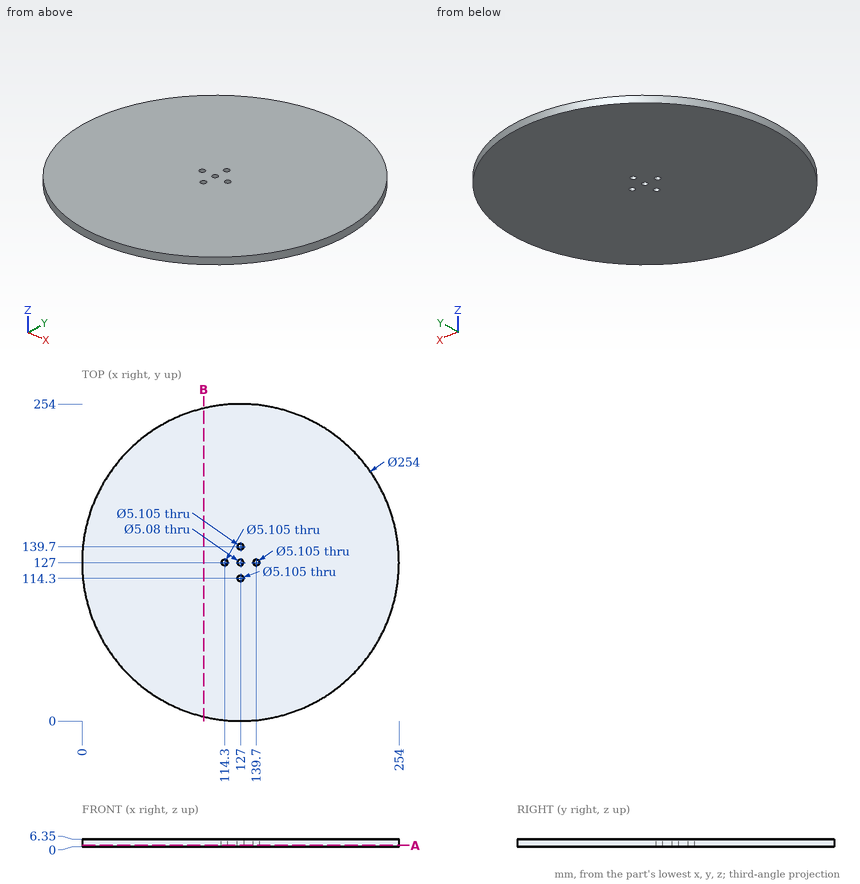
Study the drawing (mm; zero at the part's minimum x, y, z) and answer. Coordinates: 2 decimals unless noted, no trailing zeros. Loops run counter-clockwise (first coordinate to the right, second up) from the corner with the lowest first, then second, coordinate; pieces in that order, holes last. Notation, with made-up numbers: M 57,20 L 83,20 A10 ccw 83,31 Z; hole C 30,42 d1. An arc over 180 degrees is marked long. Answer in a Markdown table with one row per item.
1) Find section A-A (z = 1.25). Determine the outline of the cut face in (x, y) (1 decimal).
Answers below:
| item | result |
|---|---|
| outline | C 127,127 d254; hole C 114.3,127 d5.1; hole C 127,114.3 d5.1; hole C 127,139.7 d5.1; hole C 127,127 d5.1; hole C 139.7,127 d5.1 |
2) Given pin 1 (2 mm diameter, centred on y = 85, z = 4.5, fed in from -X); pin 2 (1 mm diameter, centred on x = 29.5, z = 4.5, fed in from -Y) (1 decimal); pin 3 (3 mm diameter, centred on y = 75, z = 2.5, fed in from +X), each flat-ended and moving along its own axis, determine where each tip first touches the part or whether it passes through.
Answers below:
| item | result |
|---|---|
| pin 1 | x = 6.8 |
| pin 2 | y = 45 |
| pin 3 | x = 243.53 |
3) Find section B-B (x = 97.5). Determine the outline of the cut face in (y, z).
Answers below:
| item | result |
|---|---|
| outline | M 3.47,0 L 250.53,0 L 250.53,6.35 L 3.47,6.35 Z |
4) Find the intervals of material crossed by probe 1 along Y at (x, z) = (127, 3); probe 2 along X at (y, z) = (114, 4.5) (1 decimal); probe 3 along X at (y, z) = (139.7, 4.5), in increasing order.
Answers below:
| item | result |
|---|---|
| probe 1 | 0 to 111.75, 116.85 to 124.46, 129.54 to 137.15, 142.25 to 254 |
| probe 2 | 0.7 to 124.5, 129.5 to 253.3 |
| probe 3 | 0.64 to 124.45, 129.55 to 253.36 |
